Autodesk Inventor part; units mm, degrees
ref_plane "YZ Plane" through (0, 0, 0) normal (1, 0, 0) x (0, 1, 0)
ref_plane "XZ Plane" through (0, 0, 0) normal (0, 1, 0) x (-1, 0, 0)
ref_plane "XY Plane" through (0, 0, 0) normal (0, 0, 1) x (1, 0, 0)
sketch "Sketch1" plane through (0, 0, 0) normal (0, 0, 1) x (1, 0, 0)
  circle A0 centre (0, 0) radius 63.5 construction
  line L0 (0, 0) -> (-110.5, 0) construction
  line L1 (-110.5, 0) -> (-110.5, -80) construction
  line L2 (0, 0) -> (189.5, 0) construction
  line L3 (189.5, 0) -> (189.5, -85) construction
  line L4 (-88, -80) -> (-63, -80) construction
  line L5 (-63, -80) -> (-63, -85) construction
  line L6 (-63, -85) -> (-88, -85) construction
  line L7 (-88, -85) -> (-88, -80) construction
  line L8 (157, -85) -> (172, -85) construction
  line L9 (172, -85) -> (172, -90) construction
  line L10 (172, -90) -> (157, -90) construction
  line L11 (157, -90) -> (157, -85) construction
  circle A1 centre (0, 0) radius 33.5 construction
  line L12 (-35.5, -80) -> (134.5, -85) construction
  line L13 (0, 0) -> (0, -63.5) construction
  line L14 (-40.8636, 0) -> (0, -58.5) construction
  line L15 (40.8636, 0) -> (0, -58.5) construction
  line L16 (-63, -80) -> (-63, -85)
  line L17 (-63, -85) -> (-88, -85)
  line L18 (-88, -85) -> (-88, -80)
  line L19 (-110.5, -80) -> (-110.5, 0)
  line L20 (-110.5, 0) -> (-40.8636, 0) construction
  line L21 (-40.8636, 0) -> (0, -58.5) construction
  line L22 (0, -58.5) -> (40.8636, 0) construction
  line L23 (40.8636, 0) -> (189.5, 0) construction
  line L24 (189.5, 0) -> (189.5, -85) construction
  line L25 (172, -85) -> (172, -90)
  line L26 (172, -90) -> (157, -90)
  line L27 (157, -90) -> (157, -85)
  line L28 (-35.5, -80) -> (-35.5, -85)
  line L29 (-35.5, -85) -> (94.5, -85)
  line L30 (40.8636, 0) -> (70.8636, 0)
  line L31 (70.8636, 0) -> (189.5, -55)
  line L32 (189.5, -55) -> (189.5, -85)
  line L33 (151, -85) -> (145, -85) construction
  line L34 (172, -85) -> (178, -85) construction
  line L35 (151, -85) -> (149, -85) construction
  line L36 (147, -85) -> (147, -70) construction
  line L37 (147, -70) -> (151, -70) construction
  line L38 (151, -70) -> (151, -85) construction
  line L39 (149, -70) -> (149, -85) construction
  line L40 (145, -78) -> (153, -78) construction
  line L41 (153, -78) -> (153, -74) construction
  line L42 (153, -74) -> (145, -74) construction
  line L43 (145, -74) -> (145, -78) construction
  line L44 (145, -78) -> (153, -74) construction
  line L45 (153, -78) -> (145, -74) construction
  line L46 (180, -85) -> (182, -85) construction
  line L47 (182, -85) -> (182, -70) construction
  line L48 (182, -70) -> (178, -70) construction
  line L49 (178, -70) -> (178, -85) construction
  line L50 (180, -70) -> (180, -85) construction
  line L51 (184, -78) -> (176, -78) construction
  line L52 (176, -78) -> (176, -74) construction
  line L53 (176, -74) -> (184, -74) construction
  line L54 (184, -74) -> (184, -78) construction
  line L55 (184, -78) -> (176, -74) construction
  line L56 (176, -78) -> (184, -74) construction
  line L57 (147, -85) -> (147, -78) construction
  line L58 (147, -85) -> (147, -78)
  line L59 (147, -78) -> (145, -78)
  line L60 (145, -78) -> (145, -74)
  line L61 (145, -74) -> (147, -74)
  line L62 (147, -74) -> (147, -70)
  line L63 (147, -70) -> (151, -70)
  line L64 (151, -70) -> (151, -74)
  line L65 (151, -74) -> (153, -74)
  line L66 (153, -74) -> (153, -78)
  line L67 (153, -78) -> (151, -78)
  line L68 (151, -78) -> (151, -85)
  line L69 (147, -85) -> (134.5, -85) construction
  line L70 (157, -85) -> (151, -85)
  line L71 (147, -85) -> (94.5, -85)
  line L72 (178, -85) -> (178, -78)
  line L73 (178, -78) -> (176, -78)
  line L74 (176, -78) -> (176, -74)
  line L75 (176, -74) -> (178, -74)
  line L76 (178, -74) -> (178, -70)
  line L77 (178, -70) -> (182, -70)
  line L78 (182, -70) -> (182, -74)
  line L79 (182, -74) -> (184, -74)
  line L80 (184, -74) -> (184, -78)
  line L81 (184, -78) -> (182, -78)
  line L82 (182, -78) -> (182, -85)
  line L83 (189.5, -85) -> (180, -85) construction
  line L84 (178, -85) -> (149, -85) construction
  line L85 (189.5, -85) -> (182, -85)
  line L86 (178, -85) -> (172, -85)
  line L87 (-98, -80) -> (-98, -65) construction
  line L88 (-98, -65) -> (-94, -65) construction
  line L89 (-94, -65) -> (-94, -80) construction
  line L90 (-55, -80) -> (-53, -80) construction
  line L91 (-53, -80) -> (-53, -65) construction
  line L92 (-53, -65) -> (-57, -65) construction
  line L93 (-57, -65) -> (-57, -80) construction
  line L94 (-96, -65) -> (-96, -80) construction
  line L95 (-55, -65) -> (-55, -80) construction
  line L96 (-100, -73) -> (-92, -73) construction
  line L97 (-92, -73) -> (-92, -69) construction
  line L98 (-92, -69) -> (-100, -69) construction
  line L99 (-100, -69) -> (-100, -73) construction
  line L100 (-100, -73) -> (-92, -69) construction
  line L101 (-92, -73) -> (-100, -69) construction
  line L102 (-51, -73) -> (-59, -73) construction
  line L103 (-59, -73) -> (-59, -69) construction
  line L104 (-59, -69) -> (-51, -69) construction
  line L105 (-51, -69) -> (-51, -73) construction
  line L106 (-51, -73) -> (-59, -69) construction
  line L107 (-59, -73) -> (-51, -69) construction
  line L108 (-98, -80) -> (-98, -73)
  line L109 (-98, -73) -> (-100, -73)
  line L110 (-100, -73) -> (-100, -69)
  line L111 (-100, -69) -> (-98, -69)
  line L112 (-98, -69) -> (-98, -65)
  line L113 (-98, -65) -> (-94, -65)
  line L114 (-94, -65) -> (-94, -69)
  line L115 (-94, -69) -> (-92, -69)
  line L116 (-92, -69) -> (-92, -73)
  line L117 (-92, -73) -> (-94, -73)
  line L118 (-94, -73) -> (-94, -80)
  line L119 (-88, -80) -> (-94, -80)
  line L120 (-98, -80) -> (-110.5, -80)
  line L121 (-57, -80) -> (-57, -73)
  line L122 (-57, -73) -> (-59, -73)
  line L123 (-59, -73) -> (-59, -69)
  line L124 (-59, -69) -> (-57, -69)
  line L125 (-57, -69) -> (-57, -65)
  line L126 (-57, -65) -> (-53, -65)
  line L127 (-53, -65) -> (-53, -69)
  line L128 (-53, -69) -> (-51, -69)
  line L129 (-51, -69) -> (-51, -73)
  line L130 (-51, -73) -> (-53, -73)
  line L131 (-53, -73) -> (-53, -80)
  line L132 (-110.5, -80) -> (-57, -80) construction
  line L133 (-55, -80) -> (-35.5, -80) construction
  line L134 (-63, -80) -> (-57, -80)
  line L135 (-53, -80) -> (-35.5, -80)
  line L136 (0, -58.5) -> (-30, -58.5) construction
  line L137 (-30, -58.5) -> (-70.8636, 0) construction
  line L138 (-110.5, 0) -> (-70.8636, 0)
  line L139 (17.4631, -33.5) -> (-47.4631, -33.5)
  line L140 (-70.8636, 0) -> (-47.4631, -33.5)
  line L141 (17.4631, -33.5) -> (40.8636, 0)
  point P0 (149, -76)
  point P1 (180, -76)
  point P2 (-96, -71)
  point P3 (-55, -71)
  dimension "d0" = 127
  dimension "d1" = 110.5
  dimension "d2" = 80
  dimension "d3" = 75
  dimension "d4" = 189.5
  dimension "d5" = 85
  dimension "d6" = 55
  dimension "d7" = 25
  dimension "d8" = 5
  dimension "d9" = 27.5
  dimension "d10" = 15
  dimension "d11" = 5
  dimension "d13" = 67
  dimension "d14" = 5
  dimension "d19" = 30
  dimension "d20" = 30
  dimension "d21" = 17.5
  dimension "d23" = 6
  dimension "d24" = 4
  dimension "d25" = 15
  dimension "d26" = 8
  dimension "d27" = 4
  dimension "d29" = 4
  dimension "d30" = 8
  dimension "d32" = 6
  dimension "d33" = 4
  dimension "d34" = 15
  dimension "d35" = 6
  dimension "d36" = 4
  dimension "d37" = 15
  dimension "d38" = 6
  dimension "d39" = 8
  dimension "d40" = 4
  dimension "d41" = 8
  dimension "d44" = 7
  dimension "d45" = 7
  dimension "d46" = 12.5
  dimension "d47" = 30
extrude "Extrusion1" add sketch "Sketch1" along normal blind 5
fillet "Fillet1" radius 10 3 edges at (40.8636, 0, 2.5) (70.8636, 0, 2.5) (189.5, -55, 2.5)
fillet "Fillet2" radius 15 1 edges at (-110.5, 0, 2.5)
fillet "Fillet3" radius 10 3 edges at (-70.8636, 0, 2.5) (-47.4631, -33.5, 2.5) (17.4631, -33.5, 2.5)
properties part number "Soporte_Ambu_Izq"
Source: CAD feature listing. Evaluate the final solid. Frame: model axes, mm. A direction names the side the tool comes from. Round coordinates to 2 decimals unless told otherwise and drop trailing zeros. Loops run counter-clockwise (first coordinate to the right, second up) from the corner with the lowest first, then second, coordinate; pieces in that order, holes last. Notation, with made-up numbers: M 67,-29 L 81,-29 A15 ccw 81,-25 Z; hole C -34.75,32.5 d2. An arc over 180 degrees is marked long. Use a Markdown table: item, result. Add a question column.
1. Cut plane B-B, the plane x = -10. Output: boundary loops of the cut face in (y, z).
2. Pull-direction query (X, two-part tool) for faces 1 (the flat face through (-88, -83, 2)), 2 (the flat face through (127.51, -26.26, 2.46)), 3 (the flat face through (-44, -80, 2)), 4 (the flat face through (37, -54, 5)); classes: +X half, -X half, draft (parallel to the pull), parting line (faces both ways), or undercut.
3. Cut plane C-C, the plane y = -43.5. Output: boundary loops of the cut face in (x, z).
4. Cut plane A-A, the plane y = -22.5. Output: boundary loops of the cut face in (x, z), and give its area (3 significant figures).
5. Contact query for flat-ended pins moving along their axis: pin 1 (2 mm diameter, centred on x = 183.5, z = 3.5, fed in from +Y); pin 2 (0.6 mm diameter, centred on x = -99.5, z = 3.5, fed in from +Y); pin 3 (2.5 mm diameter, centred on y = -86.5, z = 2.5, fed in from -X); pin 4 (2 mm diameter, centred on x = -40.5, y = -58, fed in from -Z). Output: stop coordinate, or through.
6. Set-up query: faces 5 (the cylindrical face through (-46.932, -32.336, 2.535)), 6 (the flat face through (-104, -80, 2)), 7 (the flat face through (147, -82, 2)). Return all of +Z, -Z, +X, -X, +Y, -Y with unobstructed straight access to the full face (end or side cutting, diameter ignored); none if empty.
7. Ray query, line 1 along X through (y, z) = (-77, 3.05); line 2 along Y through (x, z) = (52, 1.6); line 3 along Y through (x, z) = (-25.5, 4.4). Return the intervals inside material, ascending. Write a range as [from, to].
Solution:
| question | item | result |
|---|---|---|
| 1 | outline | M -85,0 L -33.5,0 L -33.5,5 L -85,5 Z |
| 2 | face 1 | -X half |
| 2 | face 2 | +X half |
| 2 | face 3 | undercut |
| 2 | face 4 | draft |
| 3 | outline | M -110.5,0 L 164.69,0 L 164.69,5 L -110.5,5 Z |
| 4 | outline | M -110.5,0 L -55.15,0 L -55.15,5 L -110.5,5 Z; M 25.15,0 L 119.4,0 L 119.4,5 L 25.15,5 Z |
| 4 | area | 748 mm2 |
| 5 | pin 1 | stops at y = -51.75 |
| 5 | pin 2 | stops at y = -0.46 |
| 5 | pin 3 | stops at x = 157 |
| 5 | pin 4 | stops at z = 0 |
| 6 | face 5 | +Z, -Z, +Y |
| 6 | face 6 | +Z, -Z, -X, -Y |
| 6 | face 7 | +Z, -Z, -Y |
| 7 | line 1 | x = [-110.5, -98], [-94, -57], [-53, 145], [153, 176], [184, 189.5] |
| 7 | line 2 | y = [-85, 0] |
| 7 | line 3 | y = [-85, -33.5] |
